from build123d import *

# Parameters (mm, degrees)
SKETCH1_R           = 85.725
BOSS_EXTRUDE1_DEPTH = 114.3
CUT_EXTRUDE1_DEPTH  = 152.4
SKETCH3_R           = 2.778125
CUT_EXTRUDE2_DEPTH  = 3.175
SKETCH4_R           = 5.588
CUT_EXTRUDE3_DEPTH  = 6.096


with BuildPart() as part:
    # Sketch1 → Boss-Extrude1 (new body)
    with BuildSketch(Plane(origin=(0, 0, 0), x_dir=(1, 0, 0), z_dir=(0, 1, 0))):
        Circle(SKETCH1_R)
    extrude(amount=BOSS_EXTRUDE1_DEPTH)

    # Sketch2 → Cut-Extrude1 (cut)
    with BuildSketch(Plane(origin=(0, 114.3, 0), x_dir=(1, 0, 0), z_dir=(0, 1, 0))):
        Polygon((0, -85.725), (81.83903771, -25.517592593), (151.304734273, 75.062868172), (-38.51393236, 115.934796391), (-149.339737724, 18.86396687), (-68.774879215, -104.537816407), align=None)
    extrude(amount=-CUT_EXTRUDE1_DEPTH, mode=Mode.SUBTRACT)

    # Sketch3 → Cut-Extrude2 (cut)
    with BuildSketch(Plane(origin=(40.919518855, 0, 55.621296296), x_dir=(-0.80550234, 0, 0.592592593), z_dir=(-0.592592593, 0, -0.80550234))):
        with Locations((-36.83, 95.758)):
            Circle(SKETCH3_R)
        with Locations((11.176, 95.758)):
            Circle(SKETCH3_R)
        with Locations((-36.83, 70.358)):
            Circle(SKETCH3_R)
        with Locations((11.176, 70.358)):
            Circle(SKETCH3_R)
        with Locations((-36.83, 51.308)):
            Circle(SKETCH3_R)
        with Locations((6.096, 51.308)):
            Circle(SKETCH3_R)
        with Locations((-36.83, 30.48)):
            Circle(SKETCH3_R)
        with Locations((6.096, 30.48)):
            Circle(SKETCH3_R)
    extrude(amount=-CUT_EXTRUDE2_DEPTH, mode=Mode.SUBTRACT)

    # Sketch4 → Cut-Extrude3 (cut)
    with BuildSketch(Plane(origin=(0, 0, 0), x_dir=(-1, 0, 0), z_dir=(0, -1, 0))):
        with Locations((-45.859759427, -62.336492182)):
            Circle(SKETCH4_R)
    extrude(amount=-CUT_EXTRUDE3_DEPTH, mode=Mode.SUBTRACT)


solid = part.part
Could you check a few things on this model? Use its own coordinates, in mm. A direction names the side the tool comes from. Round coordinates to 2 decimals unless told otherwise and drop trailing zeros. Write each loop counter-clockwise with the first axis right and the second up, starting at its lowest first coordinate (ties: lowest second). Pieces come first, ordered by that corner, then holes. Notation, with made-up numbers: (-32, 14.25) -> (22, 14.25) arc R14 ccw to (22, 39.25) -> close; hole circle Ø8 at (-31.75, -35). An arc over 180 degrees is marked (long way). Use a Markdown table: item, result.
1. We'd pull the mould along Z, two halves only. Please class faces 3 (the face through (50.185, 56.35, 69.5)), 4 (the face through (41, 0, 58)), 5 (the face through (33.8, 70.4, 64.8)), 6 (the face through (40.35, 57.95, 56.04)): +Z half, -Z half, draft (parallel to the pull), parting line (faces both ways), or undercut.
Answer key:
| item | result |
|---|---|
| face 3 | +Z half |
| face 4 | draft |
| face 5 | undercut |
| face 6 | -Z half |
2. If we section it at A-A (x = 42): List the corners of the cut face in (y, z) for me, then the cut area to 3 significant figures.
Answer key:
| item | result |
|---|---|
| outline | (0, 54.83) -> (114.3, 54.83) -> (114.3, 74.73) -> (0, 74.73) -> (0, 66.38) -> (6.1, 66.38) -> (6.1, 58.3) -> (0, 58.3) -> close |
| area | 2,230 mm^2 |
3. For pin 1 Ø5 at (y, z) = (40.5, 75.5) entering from +X; pin 2 Ø5 at (y, z) = (68.5, 32) entering from -X; pin 3 Ø2 at (y, z) = (33.5, 46.5) entering from +X, each with a flat end and sliding along its axis, tell me the tip position at first contact or that it passes through.
Answer key:
| item | result |
|---|---|
| pin 1 | stops at x = 44.94 |
| pin 2 | stops at x = 69.78 |
| pin 3 | stops at x = 72.65 |
4. If we section it at D-D (x = 61.5): List the corners of the cut face in (y, z) for me, then the cut area to 3 significant figures.
Answer key:
| item | result |
|---|---|
| outline | (0, 40.48) -> (114.3, 40.48) -> (114.3, 59.72) -> (0, 59.72) -> close |
| area | 2,200 mm^2 |
5. Which directions (+Z, -Z, +X, -X, +Y, -Y) give clear straight access to the entire face, cutting with the end or side of a thin tool? Please do faces 1 (the face through (72.5, 51.35, 36.33)), 2 (the face through (46.587, 3.005, 56.796)).
Answer key:
| item | result |
|---|---|
| face 1 | none |
| face 2 | -Y |
6. If we section it at B-B (y = 21.5): List the corners of the cut face in (x, z) for me (3 decimals).
Answer key:
| item | result |
|---|---|
| outline | (0, 85.725) -> (81.839, 25.518) arc R85.725 ccw to start |
7. If we section it at C-C (z = 55): List the corners of the cut face in (x, y) for me, then the cut area to 3 significant figures.
Answer key:
| item | result |
|---|---|
| outline | (41.76, 0) -> (65.76, 0) -> (65.76, 114.3) -> (41.76, 114.3) -> close |
| area | 2,740 mm^2 |
8. Please list where these lines run through material, in increasing order: probe 1 along X at (y, z) = (6, 62); probe 2 along X at (y, z) = (69, 66); probe 3 along Z at (x, y) = (23.5, 56.5).
Answer key:
| item | result |
|---|---|
| probe 1 | x = 32.25 to 40.28, 51.44 to 59.2 |
| probe 2 | x = 26.81 to 31.67, 32.17 to 54.71 |
| probe 3 | z = 68.44 to 82.44 |
